Job drawing, mm, ordinate dimensions from the low corner. One solid piece. A direction names the side the tool comes from. Round coordinates to 2 decimals unless told otherwise and drop trailing zeros. Write each loop counter-clockwise with the first axis right and the second up, starting at its lowest first coordinate (ties: lowest second). Pieces come first, ordered by that corner, then holes. Notation, with made-up numbers: M 79,27.25 L 86,27.25 A18 cw 86,51.25 Z; hole C 43.25,-19.75 d4. An arc over 180 degrees is marked long. One line per item, written item: value. Start each with the question number.
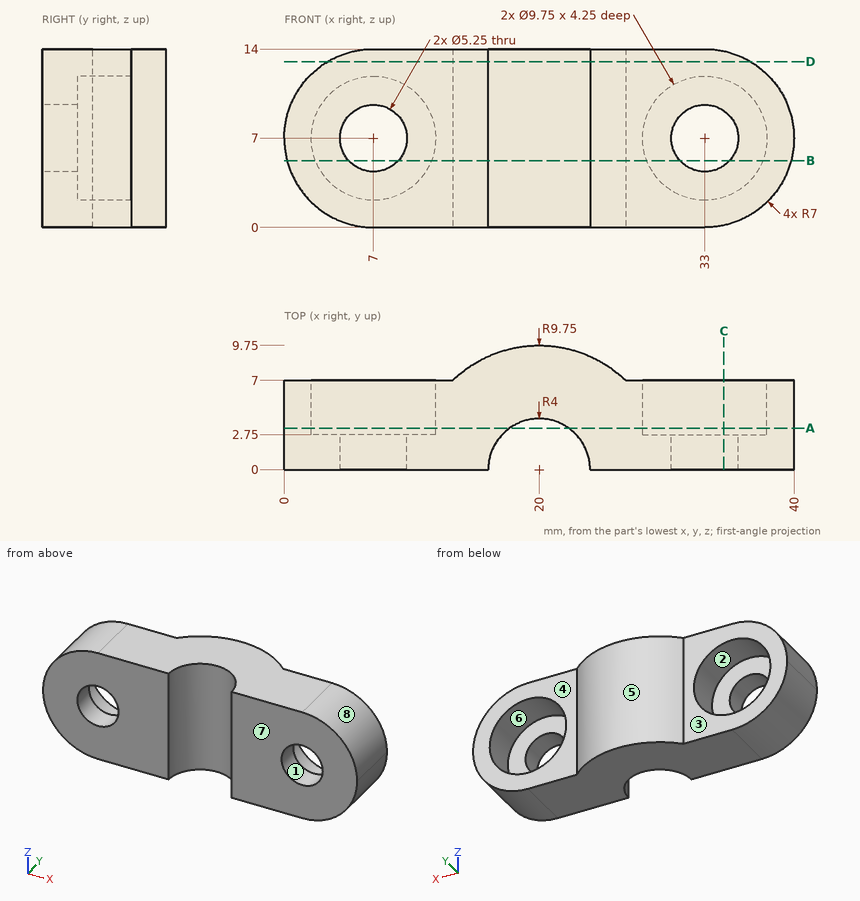
Item 1: Two-plate mould, pull along Z, no slides. Class the marked faces 6, 7 and 8: pulls with the +Z half, pulls with the -Z half, needs draft (parallel to the pull), parting line crosses it, or undercut.
Item 2: Drop flat-ended pins along their axis: pin 1 (4 mm diameter, centred on x = 21.5, z = 4, fed in from -Y); pin 2 (2 mm diameter, centred on y = 8.5, z = 4, fed in from +X); pin 3 (6.5 mm diameter, centred on x = 36.5, z = 9, fed in from +Y). Give the stop position or say it passes through.
Item 3: Drill centre lines: line 1 (X direction, y = 3.5, z = 11) (1 decimal); line 2 (X direction, y = 4.6, z = 7) (3 decimals); line 3 (Z direction, x = 33, y = 5.95) (3 decimals). Where is each one in solid material? Low to high.
Item 4: Cut at C-C, the plane x = 34.5. Write the cut outline in (y, z).
Item 5: Cut at B-B, the plane z = 5.25. Write the cut outline in (x, y), plus the area to 3 significant figures.
Item 6: Cut at D-D, the plane z = 13. Write the cut outline in (x, y), plus the area to 3 significant figures.
Item 7: Which spindle directions (+Z, -Z, +X, -X, +Y, -Y) get a long thin tool onto all of the face, cutting with end or side? Do the marked faces 1, 2, 3, 4 and 5. Say none if no direction does.
Item 8: Cut at A-A, the plane y = 3.25. Count the separate pieces of the cut face and the enclosed holes in it, plus the area to 3 significant figures.
Computed values:
1. face 6: undercut
1. face 7: needs draft
1. face 8: pulls with the +Z half
2. pin 1: stops at y = 1.94
2. pin 2: stops at x = 26.23
2. pin 3: stops at y = 7
3. line 1: x = 1.3 to 4.2, 9.8 to 18.1, 21.9 to 30.2, 35.8 to 38.7
3. line 2: x = 0 to 2.125, 11.875 to 28.125, 37.875 to 40
3. line 3: z = 0 to 2.125, 11.875 to 14
4. outline: M 0,0.16 L 7,0.16 L 7,2.36 L 2.75,2.36 L 2.75,4.85 L 0,4.85 Z; M 0,9.15 L 2.75,9.15 L 2.75,11.64 L 7,11.64 L 7,13.84 L 0,13.84 Z
5. outline: M 0.22,0 L 5.04,0 L 5.04,2.75 L 2.45,2.75 L 2.45,7 L 0.22,7 Z; M 8.96,0 L 16,0 A4 cw 24,0 L 31.04,0 L 31.04,2.75 L 28.45,2.75 L 28.45,7 L 26.79,7 A9.75 ccw 13.21,7 L 11.55,7 L 11.55,2.75 L 8.96,2.75 Z; M 34.96,0 L 39.78,0 L 39.78,7 L 37.55,7 L 37.55,2.75 L 34.96,2.75 Z
5. area: 179 mm2
6. outline: M 3.39,0 L 16,0 A4 cw 24,0 L 36.61,0 L 36.61,7 L 26.79,7 A9.75 ccw 13.21,7 L 3.39,7 Z
6. area: 233 mm2
7. face 1: +Y, -Y
7. face 2: +Y
7. face 3: +Z, -Z, -X, +Y
7. face 4: +Z, -Z, +X, +Y
7. face 5: +Z, -Z, +Y
8. separate pieces: 2
8. enclosed holes: 2
8. area: 303 mm2
